Autodesk Inventor part; units mm, degrees
ref_plane "YZ Plane" through (0, 0, 0) normal (1, 0, 0) x (0, 1, 0)
ref_plane "XZ Plane" through (0, 0, 0) normal (0, 1, 0) x (-1, 0, 0)
ref_plane "XY Plane" through (0, 0, 0) normal (0, 0, 1) x (1, 0, 0)
sketch "Sketch1" plane through (0, 0, 0) normal (0, 1, 0) x (-1, 0, 0)
  line L0 (0, 20) -> (-160, 20)
  circle A0 centre (0, -160) radius 2.5
  arc A1 (0, -180) -> (20, -160) centre (0, -160) ccw
  line L1 (0, 20) -> (-160, 20)
  arc A2 (-137.2, -66.7557) -> (-137.2, -62.7557) centre (-137.2, -64.7557) ccw
  arc A3 (-137.2, -66.7557) -> (-137.2, -62.7557) centre (-137.2, -64.7557) ccw
  line L2 (-137.2, -62.7557) -> (-163, -62.7557)
  line L3 (-137.2, -66.7557) -> (-163, -66.7557)
  arc A4 (-137.2, -100.7557) -> (-137.2, -96.7557) centre (-137.2, -98.7557) ccw
  circle A5 centre (-160, -160) radius 2.5
  circle A6 centre (-160, -160) radius 2.5
  line L4 (20, -160) -> (20, 0)
  line L5 (-180, 0) -> (-180, -160)
  line L6 (20, -160) -> (20, 0)
  line L7 (-180, 0) -> (-180, -160)
  line L8 (-160, -180) -> (0, -180)
  line L9 (-160, -180) -> (0, -180)
  arc A7 (-180, -160) -> (-160, -180) centre (-160, -160) ccw
  arc A8 (-180, -160) -> (-160, -180) centre (-160, -160) ccw
  arc A9 (-137.2, -100.7557) -> (-137.2, -96.7557) centre (-137.2, -98.7557) ccw
  arc A10 (0, -180) -> (20, -160) centre (0, -160) ccw
  circle A11 centre (0, -160) radius 2.5
  circle A12 centre (0, 0) radius 2.5
  arc A13 (20, 0) -> (0, 20) centre (0, 0) ccw
  arc A14 (20, 0) -> (0, 20) centre (0, 0) ccw
  circle A15 centre (0, 0) radius 2.5
  arc A16 (-163, -62.7557) -> (-163, -66.7557) centre (-163, -64.7557) ccw
  line L10 (-163, -96.7557) -> (-137.2, -96.7557)
  arc A17 (3, -66.7557) -> (3, -62.7557) centre (3, -64.7557) ccw
  arc A18 (3, -66.7557) -> (3, -62.7557) centre (3, -64.7557) ccw
  circle A19 centre (-160, 0) radius 2.5
  circle A20 centre (-160, 0) radius 2.5
  arc A21 (-160, 20) -> (-180, 0) centre (-160, 0) ccw
  arc A22 (-160, 20) -> (-180, 0) centre (-160, 0) ccw
  line L11 (-163, -66.7557) -> (-137.2, -66.7557)
  line L12 (-163, -100.7557) -> (-137.2, -100.7557)
  line L13 (-137.2, -100.7557) -> (-163, -100.7557)
  line L14 (-137.2, -96.7557) -> (-163, -96.7557)
  arc A23 (-163, -62.7557) -> (-163, -66.7557) centre (-163, -64.7557) ccw
  line L15 (-163, -62.7557) -> (-137.2, -62.7557)
  arc A24 (-163, -96.7557) -> (-163, -100.7557) centre (-163, -98.7557) ccw
  arc A25 (-163, -96.7557) -> (-163, -100.7557) centre (-163, -98.7557) ccw
  arc A26 (-22.8, -62.7557) -> (-22.8, -66.7557) centre (-22.8, -64.7557) ccw
  arc A27 (-22.8, -62.7557) -> (-22.8, -66.7557) centre (-22.8, -64.7557) ccw
  line L16 (-22.8, -62.7557) -> (3, -62.7557)
  line L17 (3, -62.7557) -> (-22.8, -62.7557)
  line L18 (3, -66.7557) -> (-22.8, -66.7557)
  line L19 (-22.8, -66.7557) -> (3, -66.7557)
  line L20 (-22.8, -96.7557) -> (3, -96.7557)
  line L21 (3, -96.7557) -> (-22.8, -96.7557)
  arc A28 (-22.8, -96.7557) -> (-22.8, -100.7557) centre (-22.8, -98.7557) ccw
  arc A29 (-22.8, -96.7557) -> (-22.8, -100.7557) centre (-22.8, -98.7557) ccw
  arc A30 (3, -100.7557) -> (3, -96.7557) centre (3, -98.7557) ccw
  arc A31 (3, -100.7557) -> (3, -96.7557) centre (3, -98.7557) ccw
  line L22 (3, -100.7557) -> (-22.8, -100.7557)
  line L23 (-22.8, -100.7557) -> (3, -100.7557)
  line L24 (-22.8, -66.7557) -> (3, -66.7557)
  line L25 (3, -62.7557) -> (-22.8, -62.7557)
  arc A32 (-22.8, -62.7557) -> (-22.8, -66.7557) centre (-22.8, -64.7557) ccw
  arc A33 (3, -66.7557) -> (3, -62.7557) centre (3, -64.7557) ccw
  arc A34 (20, 0) -> (0, 20) centre (0, 0) ccw
  arc A35 (20, 0) -> (0, 20) centre (0, 0) ccw
  line L26 (0, 20) -> (-160, 20)
  circle A36 centre (0, 0) radius 2.5
  circle A37 centre (0, 0) radius 2.5
  line L27 (0, 20) -> (-160, 20)
  line L28 (20, -160) -> (20, 0)
  line L29 (20, -160) -> (20, 0)
  arc A38 (0, -180) -> (20, -160) centre (0, -160) ccw
  arc A39 (0, -180) -> (20, -160) centre (0, -160) ccw
  line L30 (-66.7557, -163) -> (-66.7557, -137.2)
  line L31 (-66.7557, -137.2) -> (-66.7557, -163)
  arc A40 (-66.7557, -163) -> (-62.7557, -163) centre (-64.7557, -163) ccw
  arc A41 (-66.7557, -163) -> (-62.7557, -163) centre (-64.7557, -163) ccw
  line L32 (-96.7557, -137.2) -> (-96.7557, -163)
  line L33 (-96.7557, -163) -> (-96.7557, -137.2)
  line L34 (-100.7557, -137.2) -> (-100.7557, -163)
  line L35 (-160, -180) -> (0, -180)
  line L36 (-160, -180) -> (0, -180)
  arc A42 (-180, -160) -> (-160, -180) centre (-160, -160) ccw
  arc A43 (-100.7557, -163) -> (-96.7557, -163) centre (-98.7557, -163) ccw
  arc A44 (-180, -160) -> (-160, -180) centre (-160, -160) ccw
  arc A45 (-160, 20) -> (-180, 0) centre (-160, 0) ccw
  arc A46 (-160, 20) -> (-180, 0) centre (-160, 0) ccw
  circle A47 centre (-160, 0) radius 2.5
  circle A48 centre (-160, 0) radius 2.5
  line L37 (-180, 0) -> (-180, -160)
  line L38 (-180, 0) -> (-180, -160)
  arc A49 (-96.7557, -137.2) -> (-100.7557, -137.2) centre (-98.7557, -137.2) ccw
  circle A50 centre (-160, -160) radius 2.5
  circle A51 centre (-160, -160) radius 2.5
  arc A52 (-96.7557, -137.2) -> (-100.7557, -137.2) centre (-98.7557, -137.2) ccw
  circle A53 centre (0, -160) radius 2.5
  circle A54 centre (0, -160) radius 2.5
  line L39 (-62.7557, -163) -> (-62.7557, -137.2)
  line L40 (-62.7557, -137.2) -> (-62.7557, -163)
  arc A55 (-62.7557, -137.2) -> (-66.7557, -137.2) centre (-64.7557, -137.2) ccw
  arc A56 (-62.7557, -137.2) -> (-66.7557, -137.2) centre (-64.7557, -137.2) ccw
  line L41 (-100.7557, -163) -> (-100.7557, -137.2)
  line L42 (-96.7557, -22.8) -> (-96.7557, 3)
  line L43 (-96.7557, 3) -> (-96.7557, -22.8)
  arc A57 (-96.7557, 3) -> (-100.7557, 3) centre (-98.7557, 3) ccw
  arc A58 (-96.7557, 3) -> (-100.7557, 3) centre (-98.7557, 3) ccw
  line L44 (-100.7557, 3) -> (-100.7557, -22.8)
  arc A59 (-100.7557, -22.8) -> (-96.7557, -22.8) centre (-98.7557, -22.8) ccw
  arc A60 (-100.7557, -22.8) -> (-96.7557, -22.8) centre (-98.7557, -22.8) ccw
  line L45 (-100.7557, -22.8) -> (-100.7557, 3)
  arc A61 (-66.7557, -22.8) -> (-62.7557, -22.8) centre (-64.7557, -22.8) ccw
  line L46 (-66.7557, 3) -> (-66.7557, -22.8)
  line L47 (-66.7557, -22.8) -> (-66.7557, 3)
  arc A62 (-66.7557, -22.8) -> (-62.7557, -22.8) centre (-64.7557, -22.8) ccw
  arc A63 (-62.7557, 3) -> (-66.7557, 3) centre (-64.7557, 3) ccw
  line L48 (-62.7557, 3) -> (-62.7557, -22.8)
  line L49 (-62.7557, -22.8) -> (-62.7557, 3)
  arc A64 (-62.7557, 3) -> (-66.7557, 3) centre (-64.7557, 3) ccw
  arc A65 (-100.7557, -163) -> (-96.7557, -163) centre (-98.7557, -163) ccw
  point P0 (-22.8, -64.7557)
  point P1 (3, -64.7557)
extrude "Extrusion1" add sketch "Sketch1" along normal blind 3
properties part number "Baseprendronme"
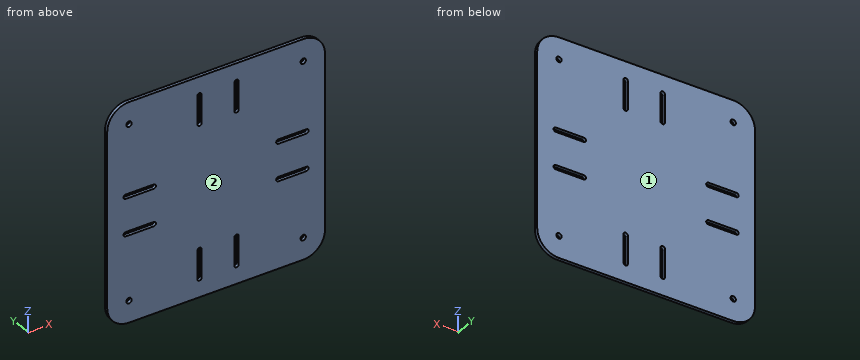
Build history of the part. All positions in model axes, mm. Face numbers are marked on the shaded views. Coordinates: 2 decimals unless noted, no trailing zeros. Write each question's results on one line, items separated by ' | '. Start each with the question number.
Item 1: Wall check: probe 1 along Z at (x, y) = (160, 0.85); probe 2 along Z at (x, y) = (153, 1.65); probe 3 along X at (y, z) = (2, -66.5). Give the ranges that are in metal, low to high. Write a range as [from, to].
Item 2: Flat gauge pin, fed straight in: pin 1 (5 mm diameter, centred on x = 151, z = -134, fed in from -Y). Where does the tip first touch, or does it go through?
Item 3: Mould opens along Y. For the marked faces 1 and 2 say: released by +Y, released by -Y, zero draft, split by the parting line, or undercut.
Numbers:
1) probe 1: [-180, -162.5], [-157.5, -100.76], [-96.76, -66.76], [-62.76, -2.5], [2.5, 20] | probe 2: [-180, -100.76], [-96.76, -66.76], [-62.76, 20] | probe 3: [-20, -3.98], [23.78, 136.22], [163.98, 180]
2) pin 1: y = 0
3) face 1: released by +Y | face 2: released by -Y
